Source: CAD feature listing. Evaluate the final solid. Frame: model axes, mm. A direction names the side the tool comes from. Coordinates: 2 decimals unless noted, no trailing zeros. Order: outer loops, then holes, each group sorted by start corner. A loop starts at its lowest first (then second) coordinate and runs counter-clockwise, first axis right, second up. Notation, with made-up numbers: (39.5, -14.75) -> (98.5, -14.75) arc R27 cw to (98.5, 22.25) -> close; hole circle Ø8 at (69, 78). An arc over 180 degrees is marked (long way). Put each result on its own line as item: value.
from build123d import *

# Parameters (mm, degrees)
F0_W     = 105
F0_H     = 55
F0_R     = 10
F1_DEPTH = 20
F3_SIZE  = 5
F4_T     = -0.6


with BuildPart() as f1:
    # F0 (on Top) → F1 (new body)
    with BuildSketch(Plane.XY):
        with Locations((52.5, 27.5)):
            Rectangle(F0_W, F0_H)
        with Locations((15, 15)):
            Circle(F0_R, mode=Mode.SUBTRACT)
        with Locations((40, 15)):
            Circle(F0_R, mode=Mode.SUBTRACT)
        with Locations((65, 15)):
            Circle(F0_R, mode=Mode.SUBTRACT)
        with Locations((90, 15)):
            Circle(F0_R, mode=Mode.SUBTRACT)
        with Locations((15, 40)):
            Circle(F0_R, mode=Mode.SUBTRACT)
        with Locations((40, 40)):
            Circle(F0_R, mode=Mode.SUBTRACT)
        with Locations((65, 40)):
            Circle(F0_R, mode=Mode.SUBTRACT)
        with Locations((90, 40)):
            Circle(F0_R, mode=Mode.SUBTRACT)
    extrude(amount=F1_DEPTH)

    # F3
    f3_edges = [f1.edges().sort_by_distance(p)[0] for p in [
        (0, 0, 10),
        (105, 0, 10),
        (105, 55, 10),
        (0, 55, 10),
    ]]
    chamfer(f3_edges, length=F3_SIZE)

    # F4
    f4_openings = [f1.faces().sort_by_distance(p)[0] for p in [
        (52.5, 27.5, 0),
    ]]
    offset(amount=F4_T, openings=f4_openings)


solid = f1.part
1. Set-up query: faces 1 (the cylindrical face through (80, 15, 10)), 2 (the flat face through (2.96, 2.89, 9.56)). Return all of +Z, -Z, +X, -X, +Y, -Y with unobstructed straight access to the full face (end or side cutting, diameter ignored); none if empty.
Numbers:
face 1: +Z, -Z
face 2: -Z
2. Cut plane B-B on x = 11. Output: boundary loops of the cut face in (y, z), plus the area to 3 significant figures.
Numbers:
outline: (0, 0) -> (0.6, 0) -> (0.6, 19.4) -> (5.18, 19.4) -> (5.18, 0) -> (5.83, 0) -> (5.83, 20) -> (0, 20) -> close; (24.17, 0) -> (24.82, 0) -> (24.82, 19.4) -> (30.18, 19.4) -> (30.18, 0) -> (30.83, 0) -> (30.83, 20) -> (24.17, 20) -> close; (49.17, 0) -> (49.82, 0) -> (49.82, 19.4) -> (54.4, 19.4) -> (54.4, 0) -> (55, 0) -> (55, 20) -> (49.17, 20) -> close
area: 84.8 mm2
3. Pull-direction query (X, two-part tool) for faces 3 (the cylindrical face through (31.59, 8.55, 9.56)), 4 (the flat face through (105, 27, 10)), 5 (the cylindrical face through (82, 34, 10)), 6 (the flat face through (3, 2, 10)); classes: pulls with the +X half, pulls with the -X half, needs draft (parallel to the pull), parting line crosses it, or undercut.
Numbers:
face 3: undercut
face 4: pulls with the +X half
face 5: undercut
face 6: pulls with the -X half
4. Cut plane A-A on z = 18. Count the separate pieces of the cut face and the enclosed holes in it, plus the area to 3 significant figures.
Numbers:
separate pieces: 9
enclosed holes: 9
area: 494 mm2
5. Ray query, line 1 along Y through (x, z) = (40, 9.25); line 2 along Y through (x, z) = (86, 8); line 3 along Z through (x, y) = (74, 31). Return the intervals inside material, ascending.
Numbers:
line 1: y = 0 to 0.6, 4.4 to 5, 25 to 25.6, 29.4 to 30, 50 to 50.6, 54.4 to 55
line 2: y = 0 to 0.6, 5.18 to 5.83, 24.17 to 24.82, 30.18 to 30.83, 49.17 to 49.82, 54.4 to 55
line 3: z = 19.4 to 20
6. Cut plane D-D on x = 65. Output: boundary loops of the cut face in (y, z), plus the area to 3 significant figures.
Numbers:
outline: (0, 0) -> (0.6, 0) -> (0.6, 19.4) -> (4.4, 19.4) -> (4.4, 0) -> (5, 0) -> (5, 20) -> (0, 20) -> close; (25, 0) -> (25.6, 0) -> (25.6, 19.4) -> (29.4, 19.4) -> (29.4, 0) -> (30, 0) -> (30, 20) -> (25, 20) -> close; (50, 0) -> (50.6, 0) -> (50.6, 19.4) -> (54.4, 19.4) -> (54.4, 0) -> (55, 0) -> (55, 20) -> (50, 20) -> close
area: 78.8 mm2
7. First-contact query: pin 1 (18 mm diameter, centred on x = 40, y = 15, fed in from -Z). Flat tip, straight axial feed; report the tip coordinate or a pass-through.
Numbers:
pin 1: passes through
